Can you work these out from the model? Positions are in its coordinate system, mm. A direction names the side the tool comes from. Round coordinates to 2 decimals unless told otherwise and drop trailing zeros. Loops run counter-clockwise (first coordinate to the right, second up) from the corner with the lowest first, then second, coordinate; pieces in that order, holes last. Notation, with made-up numbers: M -33.5,45 L -27.5,45 A14 ccw -27.5,64 Z; hole C 2.5,-26 d9. An arc over 180 degrees is marked long. Answer as CSV lines item,"result".
Autodesk Inventor part; units mm, degrees
ref_plane "YZ Plane" through (0, 0, 0) normal (1, 0, 0) x (0, 1, 0)
ref_plane "XZ Plane" through (0, 0, 0) normal (0, 1, 0) x (-1, 0, 0)
ref_plane "XY Plane" through (0, 0, 0) normal (0, 0, 1) x (1, 0, 0)
sketch "Esquisse1" plane through (0, 0, 0) normal (0, 0, 1) x (1, 0, 0)
  line L0 (0, 0) -> (0, 32) construction
  line L1 (0, 32) -> (27.7128, 16) construction
  line L2 (27.7128, 16) -> (0, 0) construction
  circle A0 centre (0, 0) radius 2
  circle A1 centre (0, 32) radius 2
  circle A2 centre (27.7128, 16) radius 2
  line L3 (0, 32) -> (0, 48) construction
  line L4 (35.7128, 48) -> (35.7128, 11.3812)
  line L5 (2.1436, -8) -> (-8, -8)
  line L6 (-8, -8) -> (-8, 48)
  line L7 (-8, 48) -> (35.7128, 48)
  line L8 (27.7128, 16) -> (35.7128, 16) construction
  line L9 (0, 0) -> (0, -8) construction
  line L10 (0, 32) -> (-8, 32) construction
  line L11 (27.7128, 16) -> (31.7128, 9.0718) construction
  line L12 (35.7128, 11.3812) -> (2.1436, -8)
  dimension "d0" = 32
  dimension "d1" = 32
  dimension "d2" = 32
  dimension "d3" = 4
  dimension "d4" = 16
  dimension "d5" = 8
  dimension "d6" = 8
  dimension "d7" = 8
  dimension "d27" = 8
extrude "Extrusion1" add sketch "Esquisse1" along normal blind 10
sketch "Esquisse2" plane through (0, 0, 0) normal (0, 0, -1) x (-1, 0, 0)
  circle A0 centre (-27.7128, 16) radius 2
  circle A1 centre (0, 32) radius 2
  circle A2 centre (0, 0) radius 2
  line L0 (-35.7128, 48) -> (-35.7128, -8)
  line L1 (8, -8) -> (8, 48)
  line L2 (8, 48) -> (-35.7128, 48)
  line L3 (0, 27.9585) -> (-3.5, 29.9793)
  line L4 (-3.5, 29.9793) -> (-3.5, 34.0207)
  line L5 (-3.5, 34.0207) -> (0, 36.0415)
  line L6 (0, 36.0415) -> (3.5, 34.0207)
  line L7 (3.5, 34.0207) -> (3.5, 29.9793)
  line L8 (3.5, 29.9793) -> (0, 27.9585)
  line L9 (-3.5, 2.0207) -> (0, 4.0415)
  line L10 (0, 4.0415) -> (3.5, 2.0207)
  line L11 (3.5, 2.0207) -> (3.5, -2.0207)
  line L12 (3.5, -2.0207) -> (0, -4.0415)
  line L13 (0, -4.0415) -> (-3.5, -2.0207)
  line L14 (-3.5, -2.0207) -> (-3.5, 2.0207)
  line L15 (-3.5, 29.9793) -> (3.5, 29.9793) construction
  line L16 (-24.2128, 13.9793) -> (-27.7128, 11.9585)
  line L17 (-27.7128, 11.9585) -> (-31.2128, 13.9793)
  line L18 (-31.2128, 13.9793) -> (-31.2128, 18.0207)
  line L19 (-31.2128, 18.0207) -> (-27.7128, 20.0415)
  line L20 (-27.7128, 20.0415) -> (-24.2128, 18.0207)
  line L21 (-24.2128, 18.0207) -> (-24.2128, 13.9793)
  point P0 (-2.1436, -8)
  dimension "d10" = 7
extrude "Extrusion2" cut sketch "Esquisse2" against normal blind 3
sketch "Esquisse5" plane through (0, 0, 0) normal (0, 0, -1) x (-1, 0, 0)
  line L0 (-35.7128, 48) -> (-35.7128, 11.3812)
  line L1 (8, -8) -> (8, 48)
  line L2 (8, 48) -> (-35.7128, 48)
  line L3 (-35.7128, 48) -> (8, 48)
  line L4 (8, 48) -> (8, 36)
  line L5 (8, 36) -> (-35.7128, 36)
  line L6 (-35.7128, 36) -> (-35.7128, 48)
  point P0 (0, 0)
  dimension "d28" = 12
extrude "Extrusion5" add sketch "Esquisse5" along normal blind 40
sketch "Esquisse6" plane through (0.0718, 36, 0) normal (0, -1, 0) x (1, 0, 0)
  line L0 (-8.0718, 0) -> (-8.0718, -40)
  line L1 (35.641, 0) -> (35.641, -40)
  line L2 (35.641, -20) -> (-8.0718, -20) construction
  circle A0 centre (35.641, -20) radius 12
  line L3 (35.641, -20) -> (35.641, -6.5) construction
  line L4 (35.641, -6.5) -> (29.141, -6.5) construction
  line L5 (29.141, -6.5) -> (21.141, -6.5) construction
  line L6 (21.141, -6.5) -> (13.141, -6.5) construction
  line L7 (13.141, -6.5) -> (5.141, -6.5) construction
  line L8 (35.641, -20) -> (-0.359, -20) construction
  line L9 (-0.359, -20) -> (-0.359, -12) construction
  circle A1 centre (-0.359, -12) radius 1
  circle A2 centre (5.141, -6.5) radius 1
  circle A3 centre (13.141, -6.5) radius 1
  circle A4 centre (21.141, -6.5) radius 1
  circle A5 centre (-0.359, -28) radius 1
  circle A6 centre (5.141, -33.5) radius 1
  circle A7 centre (13.141, -33.5) radius 1
  circle A8 centre (21.141, -33.5) radius 1
  point P0 (-0.0718, 0)
  dimension "d31" = 24
  dimension "d32" = 13.5
  dimension "d33" = 6.5
  dimension "d34" = 8
  dimension "d35" = 8
  dimension "d36" = 8
  dimension "d37" = 36
  dimension "d38" = 8
  dimension "d39" = 2
extrude "Extrusion6" cut sketch "Esquisse6" against normal through all
fillet "Congé1" radius 10 1 edges at (-8, -8, 5)
fillet "Congé2" radius 10 1 edges at (35.7128, 11.3812, 5)
fillet "Congé3" radius 10 1 edges at (2.1436, -8, 5)
fillet "Congé4" radius 10 1 edges at (-8, 42, -40)
fillet "Congé5" radius 10 1 edges at (35.7128, 42, -8)
fillet "Congé6" radius 5 1 edges at (35.7128, 42, -32)
fillet "Congé7" radius 5 1 edges at (35.7128, 42, -40)
properties part number "joint3+ax12imprint_v4"
Item 1: If we section it at D-D on y = 10.5: Write out the boundary of the cut face in (x, z).
Output:
outline,"M -8,0 L 33.18,0 L 33.18,10 L -8,10 Z"
Item 2: Will these pins go through, and if not, where does the flat tip stop? pin 1 (3.5 mm diameter, centred on y = -0.5, z = 2, fed in from +X); pin 2 (7.5 mm diameter, centred on x = 29, y = 15.5, fed in from -Z); pin 3 (3 mm diameter, centred on x = -0.29, z = -12, fed in from -Y).
Output:
pin 1,"stops at x = 18.17"
pin 2,"stops at z = 0"
pin 3,"stops at y = 36"
Item 3: We'd pull the mould along Z, two halves only. Please class faces 4 (the face through (-0.42, 41.92, -27.01)), 5 (the face through (29.487, 19.017, 1.479)), 6 (the face through (29, 14, 3)): released by +Z, released by -Z, zero draft, split by the parting line, or undercut.
Output:
face 4,"undercut"
face 5,"zero draft"
face 6,"released by -Z"
Item 4: On a 3-axis mill with a long thin cutter (end or side, diameter ignored), from which of +Z, -Z, +X, -X, +Y, -Y can I reach the whole of each face in a straight line? I mean faces 1 (the face through (17, 42, -40)), 2 (the face through (-1.726, 3.045, 1.479)), 3 (the face through (34.76, 41.92, -33.31)). Say none if no direction works.
Output:
face 1,"-Z, +X, -X, +Y, -Y"
face 2,"-Z"
face 3,"+X, +Y, -Y"
Item 5: If we section it at C-C on x = 8: Write out the boundary of the cut face in (y, z), then the cut area to 3 significant figures.
Output:
outline,"M -4.62,0 L 36,0 L 36,-40 L 48,-40 L 48,10 L -4.62,10 Z"
area,"1,010 mm2"
Item 6: If we section it at A-A on y = 39.5: State how many separate pieces and enclosed holes the cut face has, then the cut area to 3 significant figures.
Output:
separate pieces,"1"
enclosed holes,"8"
area,"1,900 mm2"
Item 7: If I drill on line 1 along Z through (x, y) = (33.5, 15); line 2 along X through (y, z) = (0, 6); line 3 along Y through (x, z) = (24, -29.5), over which ranges is the centre line in solid material (lowest first)? Write a range as from..to.
Output:
line 1,"z = 0..10"
line 2,"x = -7.38..-2, 2..16"
line 3,"y = 36..48"
Item 8: If we section it at B-B on z = -28: Write out the boundary of the cut face in (x, y).
Output:
outline,"M -8,36 L -1.29,36 L -1.29,48 L -8,48 Z; M 0.71,36 L 26.77,36 L 26.77,48 L 0.71,48 Z"
